Read the model definition and answer for the solid it produces. Units are mm, in the model's axes. A direction names the side the tool comes from. Coordinates: 2 decimals unless noted, no trailing zeros. Write each loop counter-clockwise with the first axis right and the second up, starting at its lowest first coordinate (ties: lowest second). Pieces come first, ordered by that corner, then holes. Notation, with made-up numbers: (6, -37) -> (65, -37) arc R12 ccw to (65, -25) -> close; hole circle Ø8 at (34.25, 15.5). An arc over 180 degrees is marked (long way). Use CSV: the item, a comma, the result in double quotes.
from build123d import *

# Parameters (mm, degrees)
F0_W     = 22.9585338384
F0_H     = 46.6068126261
F3_DEPTH = 25.4
F4_COUNT = 14


with BuildPart() as f1:
    # F0 (on Right) → F1 (revolve)
    with BuildSketch(Plane.YZ):
        with Locations((11.4792669192, 23.3034063131)):
            Rectangle(F0_W, F0_H)
    revolve(axis=Axis((0, 11.4792669192, 0), (0, 1, 0)))

    # F2 (on face) → F3 (cut)
    with BuildSketch(Plane(origin=(0, 22.9585338384, 0), x_dir=(-1, 0, 0), z_dir=(0, 1, 0))):
        with BuildLine():
            ThreePointArc((7.3147966582, 46.0292160808), (0.1568637228, 46.6065486487), (-7.004793259, 46.0774115437))
            Line((-7.004793259, 46.0774115437), (-5.0252592191, 35.9650850296))
            Line((-5.0252592191, 35.9650850296), (0, 35.9650850296))
            Line((0, 35.9650850296), (4.6311216429, 35.9650850296))
            Line((4.6311216429, 35.9650850296), (7.3147966582, 46.0292160808))
        make_face()
    f3 = extrude(amount=-F3_DEPTH, mode=Mode.SUBTRACT)

    # F4: F3 ×14 about axis
    f4_axis = Axis((0, 11.4792669192, 0), (0, 1, 0))
    for i in range(1, F4_COUNT):
        add(f3.rotate(f4_axis, i * 360 / F4_COUNT), mode=Mode.SUBTRACT)


solid = f1.part
1. A cutting plane is placed at A-A (x = 0.5). Give the vertices of the cut face in (y, z), and give its area (3 significant figures).
Solutions:
outline,"(0, -35.97) -> (22.96, -35.97) -> (22.96, 35.97) -> (0, 35.97) -> close"
area,"1,650 mm^2"
2. A cutting plane is placed at B-B (z = -14). Give the vertices of the cut face in (x, y).
Solutions:
outline,"(-36.85, 0) -> (36.42, 0) -> (36.42, 22.96) -> (-36.85, 22.96) -> close"
3. Each of these flat-tipped pins is pushed along its axis until it touches: pin 1 Ø5 at (x, y) = (-2, 17) entering from -Z; pin 2 Ø12 at (y, z) = (7.5, 34.5) entering from -X; pin 3 Ø4 at (x, y) = (13, 8.5) entering from +Z. Where does it stop, or does it pass through?
Solutions:
pin 1,"stops at z = -35.97"
pin 2,"stops at x = -31.66"
pin 3,"stops at z = 45.29"
4. Find the intervals of material crossed by line 1 along X through (y, z) = (5.75, -34); line 2 along Z through (x, y) = (-30.5, 5.25); line 3 along X through (y, z) = (15, 34.5), in increasing order.
Solutions:
line 1,"x = -31.12 to -22.96, -12.29 to 12.29, 22.87 to 31.48"
line 2,"z = -35.24 to -33.17, -19.44 to 19.44, 32.84 to 35.24"
line 3,"x = -31.34 to -23.3, -11.25 to 11.45, 23.33 to 31.34"
5. For a pull along X with two mould halves and no side action, classify faces 1 (the flat face through (-5.954, 11.64, 40.927)), 2 (the flat face through (-28.368, 11.64, 30.334)), 3 (the cylindrical face through (10.568, 11.64, -45.393)) as pulls with the +X half, pulls with the -X half, needs draft (parallel to the pull), parting line crosses it, or undercut.
Solutions:
face 1,"undercut"
face 2,"pulls with the -X half"
face 3,"pulls with the +X half"
6. A tool of negligible diameter and unlimited length cuts with its end or side. For faces 4 (the flat face through (-41.23, 11.64, 3.3)), 5 (the flat face through (-27.954, 11.64, 22.631)), 6 (the flat face through (-23.12, 11.64, 34.29)), 7 (the flat face through (-6.03, 11.64, -41.09)), from which of +Z, -Z, +X, -X, +Y, -Y can it reach the whole face along a straight path? Write none if from no direction.
Solutions:
face 4,"-X, +Y, -Y"
face 5,"+Y, -Y"
face 6,"+Z, +Y, -Y"
face 7,"-Z, +Y, -Y"
